Can you work these out from the model? Positions are in its coordinate system, mm. Coordinates: 2 decimals unless noted, no trailing zeros. Order: outer loops, then holes, each group sorted by start corner. A loop starts at its lowest first (then second) coordinate and runs counter-clockwise, first axis right, second up. Notation, with made-up numbers: (2.5, -22) - (48.5, -22) arc R36 ccw to (48.5, 17) - close; hole circle Ø5 at (-8.75, 23.5). An arc over 180 degrees is marked (long way). Use a Markdown table: item, result. Add a question column.
(1) For pin 1 Ø2.5 at (y, z) = (-18, 147) entering from +X; pin 2 Ø1.5 at (y, z) = (-11, 183.5) entering from +X; pin 3 Ø0.9 at (y, z) = (-17, 268.5) entering from -X, each with a flat end and sliding along its axis, tell me the tip position at first contact or that it passes through.
(2) If I drill on L1, parallel to X at y = -11.75, z = 97.5; L2, parallel to X at y = -14.25, z = 377.5; L3, parallel to Y at x = -9.5, z = 106, over which ranges is the centre line in solid material (lowest first)? Write a range as [from, to].
(3) I want a section at A-A (z = 251.5). List the corners of the cut face in (x, y) for me, and give its area (3 significant figures).
```python
from build123d import *

# Parameters (mm, degrees)
ESTRUSIONE_ESTRUSIONE1_DEPTH = 400


with BuildPart() as part:
    # Schizzo1 → Estrusione-Estrusione1 (new body)
    with BuildSketch(Plane.XY):
        with BuildLine():
            Line((-10.001211602, -16.276222172), (-7.501211602, -13.776222172))
            Line((-7.501211602, -13.776222172), (-7.501211602, -8.776222172))
            Line((-7.501211602, -8.776222172), (-8.008796188, -8.268637585))
            ThreePointArc((-8.008796188, -8.268637585), (-8.733444649, -6.695460987), (-10.306621247, -5.970812526))
            Line((-10.306621247, -5.970812526), (-10.501211602, -5.776222172))
            Line((-10.501211602, -5.776222172), (-10.501211602, -2.776222172))
            Line((-10.501211602, -2.776222172), (-10.306621247, -2.581631817))
            ThreePointArc((-10.306621247, -2.581631817), (-8.733444649, -1.856983356), (-8.008796188, -0.283806758))
            Line((-8.008796188, -0.283806758), (-7.501211602, 0.223777828))
            Line((-7.501211602, 0.223777828), (9.498788398, 0.223777828))
            Line((9.498788398, 0.223777828), (10.006372984, -0.283806758))
            ThreePointArc((10.006372984, -0.283806758), (10.731021445, -1.856983356), (12.304198043, -2.581631817))
            Line((12.304198043, -2.581631817), (12.498788398, -2.776222172))
            Line((12.498788398, -2.776222172), (12.498788398, -5.776222172))
            Line((12.498788398, -5.776222172), (12.304198043, -5.970812526))
            ThreePointArc((12.304198043, -5.970812526), (10.731021445, -6.695460987), (10.006372984, -8.268637585))
            Line((10.006372984, -8.268637585), (9.498788398, -8.776222172))
            Line((9.498788398, -8.776222172), (9.498788398, -13.776222172))
            Line((9.498788398, -13.776222172), (11.998788398, -16.276222172))
            Line((11.998788398, -16.276222172), (11.998788398, -19.314402932))
            Line((11.998788398, -19.314402932), (-10.001211602, -19.314402932))
            Line((-10.001211602, -19.314402932), (-10.001211602, -16.276222172))
        make_face()
    extrude(amount=ESTRUSIONE_ESTRUSIONE1_DEPTH)


solid = part.part
```
Answers follow:
| question | item | result |
|---|---|---|
| 1 | pin 1 | stops at x = 12 |
| 1 | pin 2 | stops at x = 9.5 |
| 1 | pin 3 | stops at x = -10 |
| 2 | L1 | x = [-7.5, 9.5] |
| 2 | L2 | x = [-7.97, 9.97] |
| 2 | L3 | y = [-19.31, -15.78], [-6.17, -2.38] |
| 3 | outline | (-10.5, -5.78) - (-10.31, -5.97) arc R2.5 cw to (-8.01, -8.27) - (-7.5, -8.78) - (-7.5, -13.78) - (-10, -16.28) - (-10, -19.31) - (12, -19.31) - (12, -16.28) - (9.5, -13.78) - (9.5, -8.78) - (10.01, -8.27) arc R2.5 cw to (12.3, -5.97) - (12.5, -5.78) - (12.5, -2.78) - (12.3, -2.58) arc R2.5 cw to (10.01, -0.28) - (9.5, 0.22) - (-7.5, 0.22) - (-8.01, -0.28) arc R2.5 cw to (-10.31, -2.58) - (-10.5, -2.78) - close |
| 3 | area | 384 mm² |
